Design review of the part built by this model. Coordinates are the model's own, in mm. Coordinates: 2 decimals unless noted, no trailing zeros. Write each loop counter-clockwise with the first axis right and the second up, starting at its lowest first coordinate (ties: lowest second). Pieces come first, ordered by that corner, then holes.
Q1. Mouldability with a two-part tool opening along Y and no side actions: class faces 1 (the cylindrical face through (7.385, 5.751, 0.394)), 2 (the flat face through (3, 7, 0)) as pulls with the +Y half, pulls with the -Y half, needs draft (parallel to the pull), parting line crosses it, or undercut.
Q2. Take a section at B-B (z = 0.35). Give the boundary of the cut face in (x, y).
Q3. Take a section at D-D (x = 8.5). Give the boundary of the cut face in (y, z).
Q4. Take a section at C-C (y = 5). Give the boundary of the cut face in (x, z), and give its area (3 significant figures).
Q5. For probe 1 along X at (y, z) = (5, 0.45); probe 2 along Y at (x, z) = (5, 0.4); probe 3 along X at (y, z) = (9.75, 0.6), list the stretches that pass through material, from the lowest coordinate up.
Q6. Take a section at A-A (x = 3.5). Give the boundary of the cut face in (y, z), and give its area (3 significant figures).
```python
from build123d import *

# Parameters (mm, degrees)
SKETCH1_W              = 9
SKETCH1_H              = 10
BOARD_DEPTH            = 0.8
SKETCH2_R              = 2.5
NON_PLATED_HOLES_DEPTH = 14.816294728
SKETCH3_R              = 0.5
PLATED_HOLES_DEPTH     = 14.816294728


with BuildPart() as part:
    # Sketch1 → BOARD (new body)
    with BuildSketch(Plane.XY):
        with Locations((5, 5)):
            Rectangle(SKETCH1_W, SKETCH1_H)
    extrude(amount=BOARD_DEPTH)

    # Sketch2 → NON-PLATED HOLES (cut, through all)
    with BuildSketch(Plane.XY):
        with Locations((5, 5)):
            Circle(SKETCH2_R)
    extrude(amount=NON_PLATED_HOLES_DEPTH, mode=Mode.SUBTRACT)

    # Sketch3 → PLATED HOLES (cut, through all)
    with BuildSketch(Plane.XY):
        with Locations((1.5, 0)):
            Circle(SKETCH3_R)
        with Locations((1.5, 10)):
            Circle(SKETCH3_R)
        with Locations((8.5, 10)):
            Circle(SKETCH3_R)
        with Locations((8.5, 0)):
            Circle(SKETCH3_R)
    extrude(amount=PLATED_HOLES_DEPTH, mode=Mode.SUBTRACT)


solid = part.part
```
Response:
1. face 1: undercut
1. face 2: needs draft
2. outline: (0.5, 0) - (1, 0) arc R0.5 cw to (2, 0) - (8, 0) arc R0.5 cw to (9, 0) - (9.5, 0) - (9.5, 10) - (9, 10) arc R0.5 cw to (8, 10) - (2, 10) arc R0.5 cw to (1, 10) - (0.5, 10) - close; hole circle Ø5 at (5, 5)
3. outline: (0.5, 0) - (9.5, 0) - (9.5, 0.8) - (0.5, 0.8) - close
4. outline: (0.5, 0) - (2.5, 0) - (2.5, 0.8) - (0.5, 0.8) - close; (7.5, 0) - (9.5, 0) - (9.5, 0.8) - (7.5, 0.8) - close
4. area: 3.20 mm2
5. probe 1: x = 0.5 to 2.5, 7.5 to 9.5
5. probe 2: y = 0 to 2.5, 7.5 to 10
5. probe 3: x = 0.5 to 1.07, 1.93 to 8.07, 8.93 to 9.5
6. outline: (0, 0) - (3, 0) - (3, 0.8) - (0, 0.8) - close; (7, 0) - (10, 0) - (10, 0.8) - (7, 0.8) - close
6. area: 4.80 mm2
